Source: three-view drawing plus pictorial views. Frame: mm from the lowest corner of the part. Coordinates: 2 decimals unless noted, no trailing zeros. Write each loop counter-clockwise with the first axis right and the second up, starting at its lowest first coordinate (ties: lowest second). Pieces come first, ordered by that corner, then holes. Notation, with made-up numbers: M 53,56 L 99,56 A35 ccw 99,88 Z; hole C -14.5,44 d6. An arc over 180 degrees is marked long. Use CSV: the item, a comma, the result in double quotes.
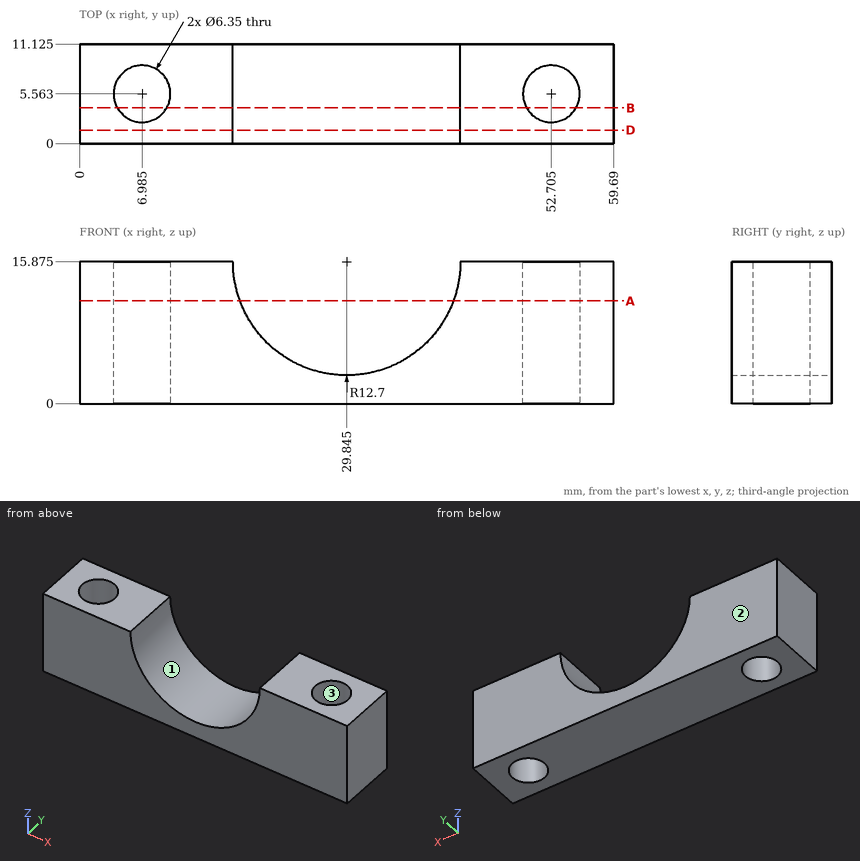
1. Mould query, pull axis Y, two halves, no side actions, for the marked faces 1, 2 and 3. Classes: pulls with the +Y half, pulls with the -Y half, needs draft (parallel to the pull), parting line crosses it, or undercut.
Resolved:
face 1,"needs draft"
face 2,"pulls with the +Y half"
face 3,"undercut"
2. Section D-D (y = 1.5). Return loops of the section in (x, z) (1 decimal), then the cut area to 3 significant figures.
Resolved:
outline,"M 0,0 L 59.7,0 L 59.7,15.9 L 42.5,15.9 A12.7 cw 17.1,15.9 L 0,15.9 Z"
area,"694 mm^2"
3. Contact query for a flat-ended pin moving along its axis: pin 1 Ø1.5 at (x, y) = (28.5, 2.5) entering from +Z. Output: stop coordinate, or through.
Resolved:
pin 1,"stops at z = 3.35"
4. Section B-B (y = 4). Return loops of the section in (x, z) (1 decimal), then the cut area to 3 significant figures.
Resolved:
outline,"M 0,0 L 4.2,0 L 4.2,15.9 L 0,15.9 Z; M 9.7,0 L 49.9,0 L 49.9,15.9 L 42.5,15.9 A12.7 cw 17.1,15.9 L 9.7,15.9 Z; M 55.5,0 L 59.7,0 L 59.7,15.9 L 55.5,15.9 Z"
area,"519 mm^2"
5. Material intervals for line 1 (X direction, y = 5, z = 1.5); line 2 (X direction, y = 5.75, z = 7.5) (1 decimal); line 3 (Y direction, x = 8, z = 3) (1 decimal), sorted ascending. Write a range as [from, to].
Resolved:
line 1,"x = [0, 3.86], [10.11, 49.58], [55.83, 59.69]"
line 2,"x = [0, 3.8], [10.2, 20.3], [39.4, 49.5], [55.9, 59.7]"
line 3,"y = [0, 2.6], [8.6, 11.1]"
6. Section A-A (z = 11.5). State how many separate pieces and enclosed holes the cut face has.
Resolved:
separate pieces,"2"
enclosed holes,"2"
